Autodesk Inventor part; units mm, degrees
ref_plane "YZ Plane" through (0, 0, 0) normal (1, 0, 0) x (0, 1, 0)
ref_plane "XZ Plane" through (0, 0, 0) normal (0, 1, 0) x (-1, 0, 0)
ref_plane "XY Plane" through (0, 0, 0) normal (0, 0, 1) x (1, 0, 0)
sketch "Sketch1" plane through (0, 0, 0) normal (0, 0, 1) x (1, 0, 0)
  line L0 (0, 0) -> (203.2, 0)
  line L1 (203.2, 0) -> (203.2, 330.2)
  line L2 (203.2, 330.2) -> (0, 330.2)
  line L3 (0, 330.2) -> (0, 0)
  dimension "d7" = 203.2
  dimension "d8" = 330.2
extrude "Extrusion1" add sketch "Sketch1" along normal blind 12.7
fillet "Fillet1" radius 6.35 8 edges at (101.6, 330.2, 0) (203.2, 165.1, 0) (203.2, 330.2, 6.35) (0, 330.2, 6.35) (101.6, 0, 0) (0, 165.1, 0) (0, 0, 6.35) (203.2, 0, 6.35)
properties material "MDF Medium Density Fiberboard"
Work out the finished part from the listing and answer in its coordinate system (mm). Coordinates: 2 decimals unless noted, no trailing zeros. Write each loop counter-clockwise with the first axis right and the second up, starting at its lowest first coordinate (ties: lowest second). Pieces come first, ordered by that corner, then holes. Notation, with made-up numbers: M -7,34 L 9,34 A20 ccw 9,60 Z; hole C -2,63 d11. An arc over 180 degrees is marked long. Write item = value, one per line.
1. A flat-ended cylindrical pin translates along its axis: pin 1 (5 mm diameter, centred on x = 33, z = 1.5, fed in from +Y). Find the tip coordinate at first contact, or state that the pin passes through.
Solution:
pin_1 = 329.75
2. Straight lines are drawn through the part: line 1 (X direction, y = 190, z = 5.75); line 2 (Y direction, x = 13, z = 6); line 3 (X direction, y = 84.5, z = 1.5). For each, find the intervals that lie inside material, in ascending order. Write a range as from..to.
Solution:
line_1 = 0.03..203.17
line_2 = 0.01..330.19
line_3 = 2.25..200.95
3. The part is cut by section A-A (z = 2.5). Determine the outline of the cut face in (x, y), then the cut area to 3 significant figures.
Solution:
outline = M 1.3,6.35 A5.05 ccw 6.35,1.3 L 196.85,1.3 A5.05 ccw 201.9,6.35 L 201.9,323.85 A5.05 ccw 196.85,328.9 L 6.35,328.9 A5.05 ccw 1.3,323.85 Z
area = 65,700 mm2
